from build123d import *

# Parameters (mm, degrees)
BOSS_EXTRUDE1_DEPTH = 10
SKETCH2_W           = 25
SKETCH2_H           = 65
CUT_EXTRUDE2_DEPTH  = 20
SKETCH3_R           = 10
CUT_EXTRUDE3_DEPTH  = 20
FILLET2_R           = 5


with BuildPart() as part:
    # Sketch1 → Boss-Extrude1 (new body)
    with BuildSketch(Plane.XY):
        with BuildLine():
            Line((-51.324273213, 15.030948404), (38.675726787, 15.030948404))
            ThreePointArc((38.675726787, 15.030948404), (51.820193251, 12.947195155), (63.675726787, 6.900266117))
            Line((63.675726787, 6.900266117), (63.675726787, -61.838369308))
            ThreePointArc((63.675726787, -61.838369308), (51.820193251, -67.885298346), (38.675726787, -69.969051596))
            Line((38.675726787, -69.969051596), (-51.324273213, -69.969051596))
            ThreePointArc((-51.324273213, -69.969051596), (-60.275029546, -69.015819954), (-68.824273213, -66.198885058))
            Line((-68.824273213, -66.198885058), (-68.824273213, 11.260781867))
            ThreePointArc((-68.824273213, 11.260781867), (-60.275029546, 14.077716763), (-51.324273213, 15.030948404))
        make_face()
    extrude(amount=BOSS_EXTRUDE1_DEPTH)

    # Sketch2 → Cut-Extrude2 (cut)
    with BuildSketch(Plane(origin=(0, 0, 0), x_dir=(-1, 0, 0), z_dir=(0, 0, -1))):
        with Locations((51.324273213, -27.469051596)):
            Rectangle(SKETCH2_W, SKETCH2_H)
    extrude(amount=-CUT_EXTRUDE2_DEPTH, mode=Mode.SUBTRACT)

    # Sketch3 → Cut-Extrude3 (cut)
    with BuildSketch(Plane(origin=(0, 0, 0), x_dir=(-1, 0, 0), z_dir=(0, 0, -1))):
        with Locations((-46.675726787, -27.469051596)):
            Circle(SKETCH3_R)
    extrude(amount=-CUT_EXTRUDE3_DEPTH, mode=Mode.SUBTRACT)

    # Fillet2
    fillet2_edges = [part.edges().sort_by_distance(p)[0] for p in [
        (51.820193251, 12.947195155, 10),
        (63.675726787, -27.469051596, 0),
        (51.820193251, -67.885298346, 0),
        (-6.324273213, 15.030948404, 10),
        (38.675726787, -69.969051596, 5),
        (-51.324273213, -69.969051596, 5),
        (-68.824273213, -66.198885058, 5),
        (-68.824273213, 11.260781867, 5),
        (-51.324273213, 15.030948404, 5),
        (38.675726787, 15.030948404, 5),
        (63.675726787, 6.900266117, 5),
        (63.675726787, -61.838369308, 5),
        (-60.275029546, 14.077716763, 10),
        (-68.824273213, -27.469051596, 10),
        (-60.275029546, -69.015819954, 10),
        (-6.324273213, -69.969051596, 10),
        (51.820193251, -67.885298346, 10),
        (63.675726787, -27.469051596, 10),
        (-6.324273213, -69.969051596, 0),
        (-60.275029546, -69.015819954, 0),
        (-68.824273213, -27.469051596, 0),
        (-60.275029546, 14.077716763, 0),
        (-6.324273213, 15.030948404, 0),
        (51.820193251, 12.947195155, 0),
    ]]
    fillet(fillet2_edges, radius=FILLET2_R - 0.0001)  # a hair under: the kernel refuses the full size


solid = part.part
Source: CAD feature listing. Evaluate the final solid. Frame: model axes, mm. A direction names the side the tool comes from. Give positions to 0.01 mm unless a question says otherwise; leave off trailing zeros. Write each loop counter-clockwise with the first axis right and the second up, starting at its lowest first coordinate (ties: lowest second). Pieces come first, ordered by that corner, then holes. Notation, with made-up numbers: (47.25, 11.5) -> (63.25, 11.5) arc R29 cw to (63.25, 34.5) -> close; hole circle Ø6 at (1, 12). An arc over 180 degrees is marked (long way). Write item = value, one per line.
Q1. Reachability of faces 1 (the face through (-63.824, -28, 5)), 2 (the face through (12, -27, 0)) from +Z, -Z, +X, -X, +Y, -Y: full face, straight path, thin tool, end or side. Return the list, or none.
Here are the results:
face_1 = +Z, -Z
face_2 = -Z, +X, -X, +Y, -Y
Q2. Mould query, pull axis Y, two halves, no side actions, for faces 3 (the face through (12, -27, 10)), 4 (the face through (-5.7, 13.6, 1.5)), 5 (the face through (-51, 5.031, 5)). Classes: +Y half, -Y half, draft (parallel to the pull), parting line (faces both ways), or undercut.
Here are the results:
face_3 = draft
face_4 = +Y half
face_5 = undercut
Q3. Cut plane D-D on y = -21. State how many separate pieces and enclosed holes the cut face has, then the cut area to 3 significant figures.
Here are the results:
separate_pieces = 3
enclosed_holes = 0
area = 901 mm²
Q4. Line query: line 1 (X direction, y = -24, z = 8); line 2 (X direction, y = -24.5, z = 6.75); line 3 (X direction, y = -11.5, z = 5.5). Output: solid intervals per line, ascending. Write a range as from..to.
Here are the results:
line_1 = -67.82..-63.82, -38.82..37.3, 56.05..62.68
line_2 = -68.51..-63.82, -38.82..37.13, 56.22..63.36
line_3 = -68.8..-63.82, -38.82..63.65
Q5. Cut plane C-C on z = 2.25. Return loops of the section in (x, y).
Here are the results:
outline = (-68, -62.82) arc R4.18 ccw to (-65.22, -66.76) arc R41.68 ccw to (-51.32, -69.14) -> (38.68, -69.14) arc R41.68 ccw to (60.9, -62.72) arc R4.18 ccw to (62.85, -59.19) -> (62.85, 4.25) arc R4.18 ccw to (60.9, 7.78) arc R41.68 ccw to (38.68, 14.21) -> (-51.32, 14.21) arc R41.68 ccw to (-65.22, 11.82) arc R4.18 ccw to (-68, 7.89) -> close; hole (-63.82, -59.97) -> (-38.82, -59.97) -> (-38.82, 5.03) -> (-63.82, 5.03) -> close; hole circle Ø20 at (46.68, -27.47)
Q6. First-contact query: pin 1 (1 mm diameter, centred on x = -12.5, z = 1.5, fed in from -Y); pin 2 (3 mm diameter, centred on x = -54, z = 4.5, fed in from -Y); pin 3 (5 mm diameter, centred on x = 26, z = 1, fed in from +Y). Flat tips, straight axial feed; report the tip coordinate or a pass-through.
Here are the results:
pin_1 = -68.97
pin_2 = -69.95
pin_3 = 14.8
